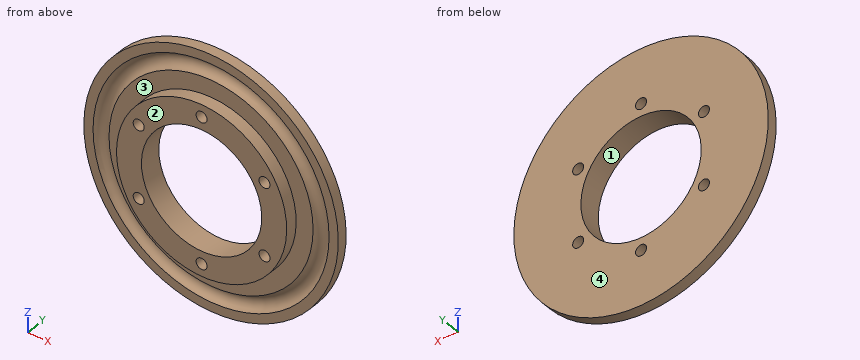
```python
from build123d import *

# Parameters (mm, degrees)
SKETCH3_R               = 24.75
BOSS_EXTRUDE1_DEPTH     = 3.6
CUT_EXTRUDE1_DEPTH      = 53.740496774
CUT_EXTRUDE1_DEPTH_BACK = 53.740496774
SKETCH4_R               = 17.5
CUT_EXTRUDE2_DEPTH      = 53.740496774
CUT_EXTRUDE2_DEPTH_BACK = 53.740496774
SKETCH5_R               = 1.6


with BuildPart() as part:
    # Sketch2 → Revolve1 (revolve)
    with BuildSketch(Plane.XY, mode=Mode.PRIVATE) as revolve1_sk:
        with BuildLine():
            Line((-34.322848467, 0), (-37, 0))
            Line((-37, 0), (-37, 3))
            Line((-37, 3), (0, 3))
            Line((0, 3), (0, 0))
            Line((0, 0), (-29.677151533, 0))
            ThreePointArc((-29.677151533, 0), (-32, 2.225), (-34.322848467, 0))
        make_face()
    revolve(revolve1_sk.sketch.rotate(Axis((0, 0, 0), (0, 1, 0)), 270), axis=Axis((0, 0, 0), (0, 1, 0)))

    # Sketch3 → Boss-Extrude1 (add)
    with BuildSketch(Plane.XZ):
        with Locations(Location((0, 0, 0), (0, 0, 90))):
            Circle(SKETCH3_R)
    extrude(amount=BOSS_EXTRUDE1_DEPTH)

    # Sketch4 → Cut-Extrude1 (cut, two sides: drawn at the far end of the back side and taken through both)
    with BuildSketch(Plane(origin=(0, 3, 0), x_dir=(1, 0, 0), z_dir=(0, 1, 0)).offset(-CUT_EXTRUDE1_DEPTH_BACK)):
        with Locations(Location((0, 0, 0), (0, 0, 270))):
            Circle(SKETCH4_R)
    extrude(amount=CUT_EXTRUDE1_DEPTH + CUT_EXTRUDE1_DEPTH_BACK, mode=Mode.SUBTRACT)

    # Sketch5 → Cut-Extrude2 (cut, two sides: drawn at the far end of the back side and taken through both)
    with BuildSketch(Plane.XZ.offset(3.6).offset(-CUT_EXTRUDE2_DEPTH_BACK)):
        with Locations(Location((-18.294786655, 10.5625, 0), (0, 0, 270))):
            Circle(SKETCH5_R)
        with Locations(Location((-18.294786655, -10.5625, 0), (0, 0, 270))):
            Circle(SKETCH5_R)
        with Locations(Location((0, -21.125, 0), (0, 0, 270))):
            Circle(SKETCH5_R)
        with Locations(Location((0, 21.125, 0), (0, 0, 270))):
            Circle(SKETCH5_R)
        with Locations(Location((18.294786655, -10.5625, 0), (0, 0, 270))):
            Circle(SKETCH5_R)
        with Locations(Location((18.294786655, 10.5625, 0), (0, 0, 270))):
            Circle(SKETCH5_R)
    extrude(amount=CUT_EXTRUDE2_DEPTH + CUT_EXTRUDE2_DEPTH_BACK, mode=Mode.SUBTRACT)


solid = part.part
```
Geometry: final body of the model. Coordinates: model frame, mm. Face numbers are marked on the shaded views. A direction names the side the tool comes from. Coordinates: 2 decimals unless noted, no trailing zeros. Order: outer loops, then holes, each group sorted by start corner. A loop starts at its lowest first (then second) coordinate and runs counter-clockwise, first axis right, second up. Notation, with made-up numbers: (71.5, -35.75) -> (116.5, -35.75) arc R21 cw to (116.5, -12.75) -> close; hole circle Ø8 at (-19, -34). An arc over 180 degrees is marked (long way). Write item = value, one per line.
(1) Pin query (flat end, axial travel): pin 1 Ø2.5 at (x, z) = (18.29, 10.56) entering from -Y. Return the tip coordinate at first contact, or that it passes through.
Solved:
pin_1 = through
(2) Pull-direction query (Z, two-part tool) for the marked faces 1 and 2; classes: pulls with the +Z half, pulls with the -Z half, needs draft (parallel to the pull), parting line crosses it, or undercut.
Solved:
face_1 = undercut
face_2 = needs draft
(3) Cut plane C-C on z = 0. Return loops of the section in (x, y) (3 decimals), plus the area to 3 significant figures.
Solved:
outline = (-37, 0) -> (-34.323, 0) arc R2.325 cw to (-29.677, 0) -> (-24.75, 0) -> (-24.75, -3.6) -> (-17.5, -3.6) -> (-17.5, 3) -> (-37, 3) -> close; (17.5, -3.6) -> (24.75, -3.6) -> (24.75, 0) -> (29.677, 0) arc R2.325 cw to (34.323, 0) -> (37, 0) -> (37, 3) -> (17.5, 3) -> close
area = 153 mm²
(4) Cut plane B-B on y = 1.25. Count the separate pieces of the cut face and the enclosed holes in it, plus the area to 3 significant figures.
Solved:
separate_pieces = 2
enclosed_holes = 8
area = 2,530 mm²
(5) Line query: line 1 (Z direction, x = -19, y = 1); line 2 (X direction, y = 0.75, z = -8); line 3 (X direction, y = 1, z = 14.5). Output: solid intervals per line, ascending.
Solved:
line_1 = -31.75 to -28.25, -23.15 to -12, -9.13 to 9.13, 12 to 23.15, 28.25 to 31.75
line_2 = -36.12 to -33.21, -28.74 to -15.56, 15.56 to 28.74, 33.21 to 36.12
line_3 = -34.04 to -30.81, -26.21 to -9.8, 9.8 to 26.21, 30.81 to 34.04
(6) Cut plane A-A on x = 0. Return loops of the section in (y, z) (3 decimals), plus the area to 3 significant figures.
Solved:
outline = (-3.6, -24.75) -> (0, -24.75) -> (0, -29.677) arc R2.325 cw to (0, -34.323) -> (0, -37) -> (3, -37) -> (3, -22.725) -> (-3.6, -22.725) -> close; (-3.6, -19.525) -> (3, -19.525) -> (3, -17.5) -> (-3.6, -17.5) -> close; (-3.6, 17.5) -> (3, 17.5) -> (3, 19.525) -> (-3.6, 19.525) -> close; (-3.6, 22.725) -> (3, 22.725) -> (3, 37) -> (0, 37) -> (0, 34.323) arc R2.325 cw to (0, 29.677) -> (0, 24.75) -> (-3.6, 24.75) -> close
area = 111 mm²
(7) Access query for the marked faces 3 and 4. Directions: +Z, -Z, +X, -X, +Y, -Y. A direction counts if a zero-diameter tool reaches every point of the face in a straight line with its end or side. Return the directions, or none.
Solved:
face_3 = -Y
face_4 = +Z, -Z, +X, -X, +Y
